For this review, take the finished solid that the model builds, in its own axes (mm). A direction names the side the tool comes from. Coordinates: 2 decimals unless noted, no trailing zeros. Loops run counter-clockwise (first coordinate to the right, second up) from the corner with the lowest first, then second, coordinate; pieces in that order, holes last.
1. Clearance check with flat-ended pins moving along their axes: P1, Ø1.7, axis at x = 26, y = 32.5, coming from the +Z side; P2, Ø5, axis at x = 30, y = 4.5, coming from the -Z side; P3, Ø3, axis at x = 20.5, y = 31.5, coming from the +Z side. State where each tip first meets the part, or that it passes through.
2. Take a section at B-B, the plane y = 28. State the section outline as (x, z) points.
3. Take a section at A-A, the plane z = 13.75. State the section outline as (x, y) points.
4. Take a section at D-D, the plane x = 38. State the section outline as (y, z) points.
5. Mouldability with a two-part tool opening along Y and no side actions: class faces 6 (the face through (29, 0, 10)), 7 (the face through (26, 3, 21.267)), 8 (the face through (34, 6.15, 21)) as pulls with the +Y half, pulls with the -Y half, needs draft (parallel to the pull), parting line crosses it, or undercut.
6. Take a section at C-C, the plane y = 16. State the section outline as (x, z) points, then the cut area to 3 significant figures.
7. Machinability: for faces 1 (the face through (40, 7.705, 16)), 2 (the face through (6.86, 17, 1)), 3 (the face through (11, 17, 5.08)), 4 (the face through (31.8, 7.5, 19.063)), 5 (the face through (4.51, 32, 23)), which of the approach directions +Z, -Z, +X, -X, +Y, -Y give a long, thin tool a straight path to every point of the face, cutting with its end or side? Answer none if there is none.
8. To check wall thickness, follow probe 1 along Y at (x, z) = (9.5, 16.5); probe 2 along X at (y, z) = (17, 9.5); probe 3 along Z at (x, y) = (33, 11). State the ranges of each line that lie inside material, in increasing order.
```python
from build123d import *

# Parameters (mm, degrees)
F0_W      = 59.5793165267
F0_H      = 34.6220657229
F1_DEPTH  = 25.4
F3_R      = 5.5412544658
F4_DEPTH  = 25.401
F5_W      = 27.6657380164
F5_H      = 19.280704204
F5_R      = 5.5412544658
F6_DEPTH  = 12.7
F8_DEPTH  = 34.6230657229
F9_W      = 16.0899236798
F9_H      = 3.0700527132
F9_W_2    = 34.4220511615
F9_H_2    = 2.5833016261
F10_DEPTH = 34.6230657229
F11_W     = 13.3519666269
F11_H     = 6.0501107946
F12_DEPTH = 59.5803165267
F2_R      = 5.219783031
F14_DEPTH = 7.62
F13_R     = 5.219783031
F15_DEPTH = 20.32
F16_R     = 2.54


with BuildPart() as f1:
    # F0 (on Top) → F1 (new body)
    with BuildSketch(Plane.XY):
        with Locations((29.7896582633, 17.3110328615)):
            Rectangle(F0_W, F0_H)
    extrude(amount=F1_DEPTH)

    # F3 (on face) → F4 (cut, through all)
    with BuildSketch(Plane.XY.offset(25.4)):
        with Locations((44.1531315446, 17.2270387411)):
            Circle(F3_R)
    extrude(amount=-F4_DEPTH, mode=Mode.SUBTRACT)

    # F5 (on face) → F6 (cut)
    with BuildSketch(Plane.XY.offset(25.4)):
        with Locations((45.7464475185, 17.3452093732)):
            Rectangle(F5_W, F5_H)
        with Locations((44.1531315446, 17.2270387411)):
            Circle(F5_R, mode=Mode.SUBTRACT)
    extrude(amount=-F6_DEPTH, mode=Mode.SUBTRACT)

    # F7 (on face) → F8 (cut, through all)
    with BuildSketch(Plane.XZ):
        Polygon((59.5793165267, 25.4), (34.7196712036, 25.4), (59.5793165267, 7.1992731339), align=None)
    extrude(amount=-F8_DEPTH, mode=Mode.SUBTRACT)

    # F9 (on face) → F10 (cut, through all)
    with BuildSketch(Plane.XZ):
        Polygon((28.0164182186, 25.4), (4.5102257282, 25.4), (4.5102257282, 21.2667640299), (8.5027217865, 21.2667640299), (24.5926454663, 21.2667640299), (28.0164182186, 21.2667640299), align=None)
        with Locations((16.5476836264, 19.7317376733)):
            Rectangle(F9_W, F9_H)
        with Locations((24.0708049387, 1.2916508131)):
            Rectangle(F9_W_2, F9_H_2)
    extrude(amount=-F10_DEPTH, mode=Mode.SUBTRACT)

    # F11 (on face) → F12 (cut, through all)
    with BuildSketch(Plane(origin=(0, 0, 0), x_dir=(0, -1, 0), z_dir=(-1, 0, 0))):
        Polygon((-6.1496212147, 25.4), (-28.8896895945, 25.4), (-28.8896895945, 19.0630443394), (-24.2999512702, 19.0630443394), (-10.9479846433, 19.0630443394), (-6.1496212147, 19.0630443394), align=None)
        with Locations((-17.6239679568, 16.0379889421)):
            Rectangle(F11_W, F11_H)
    extrude(amount=-F12_DEPTH, mode=Mode.SUBTRACT)

    # F2 (on face) → F14 (cut)
    with BuildSketch(Plane.XY.offset(25.4)):
        with Locations((10.909142904, 17.2067172825)):
            Circle(F2_R)
    extrude(amount=-F14_DEPTH, mode=Mode.SUBTRACT)

    # F13 (on face) → F15 (cut)
    with BuildSketch(Plane.XY.offset(25.4)):
        with Locations((10.909142904, 17.2067172825)):
            Circle(F13_R)
    extrude(amount=-F15_DEPTH, mode=Mode.SUBTRACT)

    # F16
    f16_edges = [f1.edges().sort_by_distance(p)[0] for p in [
        (0, 0, 12.7),
        (59.579317, 0, 3.599637),
        (59.579317, 34.622066, 3.599637),
        (0, 34.622066, 12.7),
    ]]
    fillet(f16_edges, radius=F16_R)


solid = f1.part
```
Results list:
1. P1: stops at z = 21.27
1. P2: stops at z = 2.58
1. P3: stops at z = 18.2
2. outline: (0, 0) - (6.86, 0) - (6.86, 2.58) - (41.28, 2.58) - (41.28, 0) - (59.58, 0) - (59.58, 7.2) - (43.38, 19.06) - (24.59, 19.06) - (24.59, 18.2) - (8.5, 18.2) - (8.5, 19.06) - (0, 19.06) - close
3. outline: (0, 2.54) arc R2.54 ccw to (2.54, 0) - (50.63, 0) - (50.63, 7.7) - (31.91, 7.7) - (31.91, 10.95) - (0, 10.95) - close; (0, 24.3) - (31.91, 24.3) - (31.91, 26.99) - (50.63, 26.99) - (50.63, 34.62) - (2.54, 34.62) arc R2.54 ccw to (0, 32.08) - close
4. outline: (0, 2.58) - (34.62, 2.58) - (34.62, 23) - (28.89, 23) - (28.89, 19.06) - (26.99, 19.06) - (26.99, 12.7) - (7.7, 12.7) - (7.7, 19.06) - (6.15, 19.06) - (6.15, 23) - (0, 23) - close
5. face 6: pulls with the -Y half
5. face 7: needs draft
5. face 8: undercut
6. outline: (0, 0) - (6.86, 0) - (6.86, 2.58) - (38.75, 2.58) - (38.75, 12.7) - (31.91, 12.7) - (31.91, 13.01) - (15.99, 13.01) - (15.99, 5.08) - (5.83, 5.08) - (5.83, 13.01) - (0, 13.01) - close; (49.56, 0) - (59.58, 0) - (59.58, 7.2) - (52.07, 12.7) - (49.56, 12.7) - close
6. area: 446 mm2
7. face 1: +Z, +X
7. face 2: -Z, +Y, -Y
7. face 3: +Z
7. face 4: +Z, +X, -X
7. face 5: +Z, +Y, -Y
8. probe 1: y = 0 to 10.95, 24.3 to 34.62
8. probe 2: x = 0 to 5.69, 16.12 to 38.62, 49.69 to 56.44
8. probe 3: z = 2.58 to 12.7
